Build history of the part. All positions in model axes, mm. Face numbers are marked on the shaded views. A direction names the side the tool comes from. Round coordinates to 2 decimals unless told otherwise and drop trailing zeros. Write each loop counter-clockwise with the first axis right and the second up, starting at its lowest first coordinate (ties: lowest second). Pieces come first, ordered by that corner, then holes. Notation, with made-up numbers: (88.25, 33.25) -> (117.25, 33.25) arc R17 cw to (117.25, 37.25) -> close; hole circle Ø11 at (16, 9.25). An arc over 180 degrees is marked (long way). Return JSON: item names as keys, results as strings.
Autodesk Inventor part; units mm, degrees
ref_plane "YZ Plane" through (0, 0, 0) normal (1, 0, 0) x (0, 1, 0)
ref_plane "XZ Plane" through (0, 0, 0) normal (0, 1, 0) x (-1, 0, 0)
ref_plane "XY Plane" through (0, 0, 0) normal (0, 0, 1) x (1, 0, 0)
sketch "Sketch1" plane through (0, 0, 0) normal (0, 0, 1) x (1, 0, 0)
  line L0 (-1.2233, 5.2741) -> (11.6799, 5.2741)
  line L1 (11.6799, 5.2741) -> (11.6799, -8.0863)
  line L2 (11.6799, -8.0863) -> (-1.2233, -8.0863)
  line L3 (-1.2233, -8.0863) -> (-1.2233, 5.2741)
  point P0 (0, 0)
  dimension "d0" = 12.9032
  dimension "d1" = 13.3604
extrude "Extrusion1" add sketch "Sketch1" along normal blind 6.858
sketch "Sketch2" plane through (-1.2233, 5.2741, 0) normal (0, 1, 0) x (1, 0, 0)
  circle A0 centre (6.5644, -3.3352) radius 3.2291
  line L0 (12.9032, 0) -> (12.9032, -6.858)
  point P0 (1.2233, 0)
  dimension "d4" = 6.3388
extrude "Extrusion2" add sketch "Sketch2" along normal blind 8.509
sketch "Sketch3" plane through (5.3411, 13.7831, 3.3352) normal (0, 1, 0) x (1, 0, 0)
  circle A0 centre (0, 0) radius 1.2757
  point P0 (-5.3411, 3.3352)
extrude "Extrusion3" add sketch "Sketch3" along normal blind 9.9822
properties part number "RTS Switch"
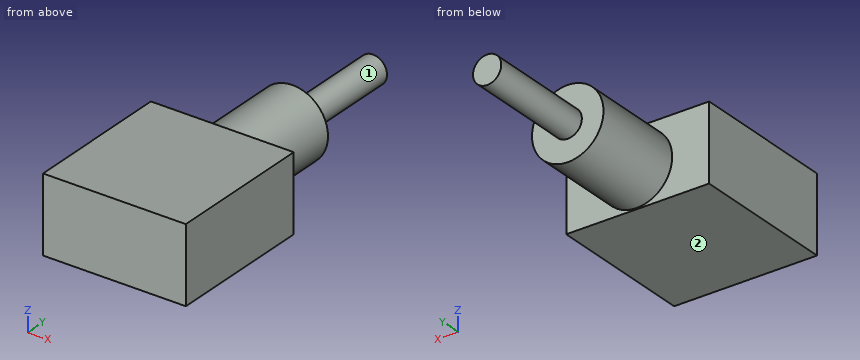
Q1. Pin check, flat tips, straight feed: pin 1 Ø4 at (y, z) = (17, 1.5) entering from +X; pin 2 Ø5 at (x, y) = (7.5, 16.5) entering from +Z. Stop position of each tip, or through.
Verdict:
{"pin 1": "stops at x = 6.62", "pin 2": "stops at z = 4.61"}
Q2. 3-axis set-ups, long thin cutter, end or side, ignore diameter. For the marked faces 1 and 2: which of +Z, -Z, +X, -X, +Y, -Y reach the whole face in a straight line?
Verdict:
{"face 1": "+Y", "face 2": "-Z, +X, -X, +Y, -Y"}
Q3. Saw through at A-A on z = 5. List the corners of the cut face in (x, y).
Verdict:
{"outline": "(-1.22, -8.09) -> (11.68, -8.09) -> (11.68, 5.27) -> (8.11, 5.27) -> (8.11, 13.78) -> (2.57, 13.78) -> (2.57, 5.27) -> (-1.22, 5.27) -> close"}
Q4. Saw through at C-C on z = 2.5. List the corners of the cut face in (x, y).
Verdict:
{"outline": "(-1.22, -8.09) -> (11.68, -8.09) -> (11.68, 5.27) -> (8.46, 5.27) -> (8.46, 13.78) -> (6.31, 13.78) -> (6.31, 23.77) -> (4.38, 23.77) -> (4.38, 13.78) -> (2.22, 13.78) -> (2.22, 5.27) -> (-1.22, 5.27) -> close"}
Q5. Saw through at D-D on y = 13.5. List the corners of the cut face in (x, z).
Verdict:
{"outline": "circle Ø6.46 at (5.34, 3.34)"}
Q6. Wall check: L1, parallel to Y at x = 3.25, z = 2.5; L2, parallel to Y at x = 8, z = 1; L3, parallel to X at y = 7, z = 3.25. Give the ranges that are in metal, low to high.
Verdict:
{"L1": "y = -8.09 to 13.78", "L2": "y = -8.09 to 5.27", "L3": "x = 2.11 to 8.57"}
Q7. Saw through at B-B on x = 5. List the corners of the cut face in (y, z), then the cut area to 3 significant figures.
Verdict:
{"outline": "(-8.09, 0) -> (5.27, 0) -> (5.27, 0.12) -> (13.78, 0.12) -> (13.78, 2.11) -> (23.77, 2.11) -> (23.77, 4.56) -> (13.78, 4.56) -> (13.78, 6.55) -> (5.27, 6.55) -> (5.27, 6.86) -> (-8.09, 6.86) -> close", "area": "171 mm²"}
